```python
from build123d import *

# Parameters (mm, degrees)
ESQUISSE1_W             = 128
ESQUISSE1_H             = 30
BOSS_EXTRU_1_DEPTH      = 10
ESQUISSE2_R             = 2
ESQUISSE2_W             = 42
ESQUISSE2_H             = 21
ENL_V_MAT_EXTRU_1_DEPTH = 10
CONG_1_R                = 5
ESQUISSE4_R             = 2.25
ENL_V_MAT_EXTRU_2_DEPTH = 10


with BuildPart() as part:
    # Esquisse1 → Boss.-Extru.1 (new body)
    with BuildSketch(Plane.XY):
        with Locations((64, 15)):
            Rectangle(ESQUISSE1_W, ESQUISSE1_H)
    extrude(amount=BOSS_EXTRU_1_DEPTH)

    # Esquisse2 → Enlèv. mat.-Extru.1 (cut)
    with BuildSketch(Plane(origin=(0, 0, 0), x_dir=(-1, 0, 0), z_dir=(0, 0, -1))):
        with Locations((-121, 10)):
            Circle(ESQUISSE2_R)
        with Locations((-121, 20)):
            Circle(ESQUISSE2_R)
        with Locations((-72, 10)):
            Circle(ESQUISSE2_R)
        with Locations((-72, 20)):
            Circle(ESQUISSE2_R)
        with Locations((-97, 15)):
            Rectangle(ESQUISSE2_W, ESQUISSE2_H)
    extrude(amount=-ENL_V_MAT_EXTRU_1_DEPTH, mode=Mode.SUBTRACT)

    # Congé1
    cong_1_edges = [part.edges().sort_by_distance(p)[0] for p in [
        (128, 30, 5),
        (128, 0, 5),
    ]]
    fillet(cong_1_edges, radius=CONG_1_R)

    # Esquisse4 → Enlèv. mat.-Extru.2 (cut)
    with BuildSketch(Plane.XY.offset(10)):
        with Locations((15, 23)):
            Circle(ESQUISSE4_R)
        with Locations((15, 7)):
            Circle(ESQUISSE4_R)
    extrude(amount=-ENL_V_MAT_EXTRU_2_DEPTH, mode=Mode.SUBTRACT)


solid = part.part
```
Here's how the part is built. I have some questions about the finished solid (model axes, mm). A direction names the side the tool comes from. Round coordinates to 2 decimals unless told otherwise and drop trailing zeros. Order: outer loops, then holes, each group sorted by start corner. A loop starts at its lowest first (then second) coordinate and runs counter-clockwise, first axis right, second up. Notation, with made-up numbers: M 46,70 L 54,70 A19 cw 54,98 Z; hole C 70.5,89 d10. An arc over 180 degrees is marked long. Answer as CSV lines item,"result".
Item 1: For pin 1 (3 mm diameter, centred on x = 72, y = 10, fed in from -Z), with a flat end and sliding along its axis, tell me the tip position at first contact or that it passes through.
From the geometry:
pin 1,"through"
Item 2: Imagine slicing it at B-B on x = 92. List the corners of the cut face in (y, z) for me, and give its area (3 significant figures).
From the geometry:
outline,"M 0,0 L 4.5,0 L 4.5,10 L 0,10 Z; M 25.5,0 L 30,0 L 30,10 L 25.5,10 Z"
area,"90.0 mm2"
Item 3: We'd pull the mould along X, two halves only. Please class faces 1 (the flat face through (61, 30, 5)), 2 (the cylindrical face through (123, 20, 5)), 3 (the flat face through (0, 15, 5)): +X half, -X half, draft (parallel to the pull), parting line (faces both ways), or undercut.
From the geometry:
face 1,"draft"
face 2,"undercut"
face 3,"-X half"
Item 4: Please list where these lines run through material, in increasing order: L1, parallel to Y at x = 15, z = 5.75; L2, parallel to Y at x = 72, z = 3.5; L3, parallel to Y at x = 90, z = 1.5. Write a range as [from, to].
From the geometry:
L1,"[0, 4.75], [9.25, 20.75], [25.25, 30]"
L2,"[0, 8], [12, 18], [22, 30]"
L3,"[0, 4.5], [25.5, 30]"
Item 5: Imagine slicing it at A-A on x = 72. List the corners of the cut face in (y, z) for me.
From the geometry:
outline,"M 0,0 L 8,0 L 8,10 L 0,10 Z; M 12,0 L 18,0 L 18,10 L 12,10 Z; M 22,0 L 30,0 L 30,10 L 22,10 Z"
Item 6: Imagine slicing it at C-C on z = 6. List the corners of the cut face in (x, y) for me, and give its area (3 significant figures).
From the geometry:
outline,"M 0,0 L 123,0 A5 ccw 128,5 L 128,25 A5 ccw 123,30 L 0,30 Z; hole C 15,7 d4.5; hole C 15,23 d4.5; hole C 72,10 d4; hole C 72,20 d4; hole M 76,4.5 L 118,4.5 L 118,25.5 L 76,25.5 Z; hole C 121,10 d4; hole C 121,20 d4"
area,"2,870 mm2"
Item 7: Which directions (+Z, -Z, +X, -X, +Y, -Y) give clear straight access to the entire face, cutting with the end or side of a thin tool? Please do faces 4 (the flat face through (49, 15, 10)), 5 (the flat face through (97, 4.5, 5)).
From the geometry:
face 4,"+Z, +X, -X, +Y, -Y"
face 5,"+Z, -Z"
